Autodesk Inventor part; units mm, degrees
ref_plane "YZ Plane" through (0, 0, 0) normal (1, 0, 0) x (0, 1, 0)
ref_plane "XZ Plane" through (0, 0, 0) normal (0, 1, 0) x (-1, 0, 0)
ref_plane "XY Plane" through (0, 0, 0) normal (0, 0, 1) x (1, 0, 0)
sketch "Sketch1" plane through (0, 0, 0) normal (0, 0, 1) x (1, 0, 0)
  circle A0 centre (0, -59.15) radius 57.15
  circle A1 centre (0, -59.15) radius 59.15
  circle A2 centre (0, -59.15) radius 55.15
  point P0 (0, 0)
  dimension "d0" = 110.3
extrude "Extrusion1" add sketch "Sketch1" along normal blind 500 contours A0
sketch "Sketch2" plane through (0, 0, 0) normal (1, 0, 0) x (0, 1, 0)
  line L0 (-2, 500) -> (-116.3, 500)
  line L1 (-2, 0) -> (-116.3, 0)
  line L2 (-2, 500) -> (-116.3, 500)
  line L3 (-2, 500) -> (-116.3, 500)
  line L4 (-116.3, 500) -> (-116.3, 350)
  line L5 (-116.3, 350) -> (-2, 350)
  line L6 (-2, 350) -> (-2, 500)
  point P0 (0, 0)
  dimension "d3" = 114.3
  dimension "d4" = 150
extrude "Extrusion2" cut sketch "Sketch2" along normal blind 500
properties part number "4.5 inch diameter pipe"
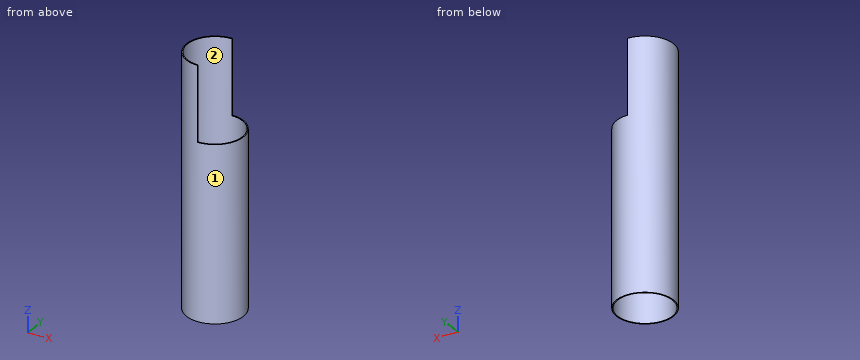
Input: part model. Units: mm. Frame: model coordinates. Face numbers are marked on the shaded views. Coordinates: 2 decimals unless noted, no trailing zeros. Order: outer loops, then holes, each group sorted by start corner. A loop starts at its lowest first (then second) coordinate and runs counter-clockwise, first axis right, second up. Notation, with made-up numbers: (76, 0.5) - (121, 0.5) arc R16 ccw to (121, 7.5) - close; hole circle Ø5 at (57, 59). An arc over 180 degrees is marked (long way). Return JSON: item names as keys, results as strings.
Q1. Ray query, probe 1 along Y at (x, z) = (0, 173); probe 2 along X at (y, z) = (-59, 250); probe 3 along Y at (x, z) = (-28, 102.5). Return the intervals inside material, ascending.
The answers:
{"probe 1": "y = -116.3 to -114.3, -4 to -2", "probe 2": "x = -57.15 to -55.15, 55.15 to 57.15", "probe 3": "y = -108.97 to -106.66, -11.64 to -9.33"}
Q2. Cut plane C-C (z = 239). Return loops of the section in (x, y), then the cut area to 3 significant figures.
The answers:
{"outline": "circle Ø114.3 at (0, -59.15); hole circle Ø110.3 at (0, -59.15)", "area": "706 mm2"}
Q3. Cut plane A-A (y = -59.15). Return loops of the section in (x, z), then the cut area to 3 significant figures.
The answers:
{"outline": "(-57.15, 0) - (-55.15, 0) - (-55.15, 500) - (-57.15, 500) - close; (55.15, 0) - (57.15, 0) - (57.15, 350) - (55.15, 350) - close", "area": "1,700 mm2"}
Q4. First-contact query: pin 1 (6 mm diameter, centred on y = -61.5, z = 439, fed in from +X); pin 2 (8 mm diameter, centred on y = -56.5, z = 147, fed in from -X); pin 3 (12 mm diameter, centred on x = 43, y = -75, fed in from -Z); pin 4 (6 mm diameter, centred on y = -23, z = 130.5, fed in from +X). Flat tips, straight axial feed; report the tip coordinate or a pass-through.
The answers:
{"pin 1": "stops at x = -54.89", "pin 2": "stops at x = -57.15", "pin 3": "passes through", "pin 4": "stops at x = 46.55"}
Q5. Cut plane D-D (z = 363). Return loops of the section in (x, y).
The answers:
{"outline": "(0, -116.3) - (0, -114.3) arc R55.15 cw to (0, -4) - (0, -2) arc R57.15 ccw to start"}
Q6. Draft query along X for the marked faces 1 and 2. Return one class per face: +X half, -X half, draft (parallel to the pull), parting line (faces both ways), or undercut.
The answers:
{"face 1": "parting line", "face 2": "undercut"}
Q7. Cut plane B-B (x = -48.5). Return loops of the section in (y, z), then the cut area to 3 significant figures.
The answers:
{"outline": "(-89.38, 0) - (-85.4, 0) - (-85.4, 500) - (-89.38, 500) - close; (-32.9, 0) - (-28.92, 0) - (-28.92, 500) - (-32.9, 500) - close", "area": "3,980 mm2"}
